```python
from build123d import *

# Parameters (mm, degrees)
IZIM1_R                     = 3
Y_KSEKLIK_EKSTR_ZYON1_DEPTH = 3.5
PAH1_SIZE                   = 0.25


with BuildPart() as part:
    # Çizim1 → Yükseklik-Ekstrüzyon1 (new body)
    with BuildSketch(Plane.XY):
        Polygon((5.196152423, 0), (2.598076211, 4.5), (-2.598076211, 4.5), (-5.196152423, 0), (-2.598076211, -4.5), (2.598076211, -4.5), align=None)
        Circle(IZIM1_R, mode=Mode.SUBTRACT)
    extrude(amount=Y_KSEKLIK_EKSTR_ZYON1_DEPTH)

    # Pah1
    pah1_edges = [part.edges().sort_by_distance(p)[0] for p in [
        (-3, 0, 0),
        (-3, 0, 3.5),
    ]]
    chamfer(pah1_edges, length=PAH1_SIZE)


solid = part.part
```
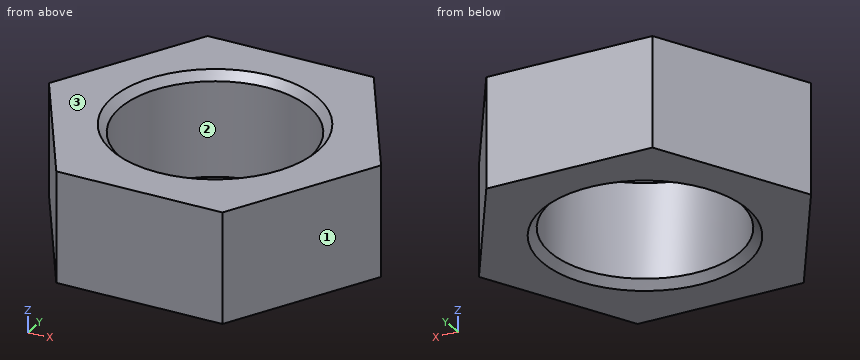
Build history of the part. All positions in model axes, mm. Face numbers are marked on the shaded views. Round coordinates to 2 decimals unless told otherwise and drop trailing zeros. Write each loop counter-clockwise with the first axis right and the second up, starting at its lowest first coordinate (ties: lowest second). Pieces come first, ordered by that corner, then holes. Notation, with made-up numbers: (44, 10.5) - (61, 10.5) arc R25 cw to (61, 27.5) - close; hole circle Ø2 at (32, 66). An arc over 180 degrees is marked (long way). Answer as CSV lines item,"result".
Q1. Drill centre lines: probe 1 along Y at (x, z) = (0, 1.4); probe 2 along Y at (x, z) = (2, 2.55); probe 3 along X at (y, z) = (-1.5, 1.15). Where is each one in solid material? Low to high. Write a range as [from, to].
Report:
probe 1,"y = [-4.5, -3], [3, 4.5]"
probe 2,"y = [-4.5, -2.24], [2.24, 4.5]"
probe 3,"x = [-4.33, -2.6], [2.6, 4.33]"
Q2. Cut at B-B (z = 2.3). Write the cut outline in (x, y).
Report:
outline,"(-5.2, 0) - (-2.6, -4.5) - (2.6, -4.5) - (5.2, 0) - (2.6, 4.5) - (-2.6, 4.5) - close; hole circle Ø6 at (0, 0)"
Q3. Cut at A-A (x = 0). Write the cut outline in (y, z), and give its area (3 significant figures).
Report:
outline,"(-4.5, 0) - (-3.25, 0) - (-3, 0.25) - (-3, 3.25) - (-3.25, 3.5) - (-4.5, 3.5) - close; (3, 0.25) - (3.25, 0) - (4.5, 0) - (4.5, 3.5) - (3.25, 3.5) - (3, 3.25) - close"
area,"10.4 mm^2"
Q4. Pull direction X, two halves, no side cores. Call the marked faces 1, 2 and 3: +X half, -X half, draft (parallel to the pull), parting line (faces both ways), or undercut.
Report:
face 1,"+X half"
face 2,"undercut"
face 3,"draft"
Q5. Cut at C-C (x = -3.5). Write the cut outline in (y, z), and give its area (3 significant figures).
Report:
outline,"(-2.94, 0) - (2.94, 0) - (2.94, 3.5) - (-2.94, 3.5) - close"
area,"20.6 mm^2"
